from build123d import *

# Parameters (mm, degrees)
SKETCH_1_W          = 58.5
SKETCH_1_H          = 60
EXTRUDE_1_DEPTH     = 1.5
FILLET_1_R          = 2.5
CUT_EXTRUDE_1_DEPTH = 2.5


with BuildPart() as part:
    # Эскиз1 → Бобышка-Вытянуть1 (new body)
    with BuildSketch(Plane.XY):
        with Locations((29.25, 30)):
            Rectangle(SKETCH_1_W, SKETCH_1_H)
    extrude(amount=EXTRUDE_1_DEPTH)

    # Скругление1
    fillet_1_edges = [part.edges().sort_by_distance(p)[0] for p in [
        (58.5, 0, 0.75),
        (0, 0, 0.75),
    ]]
    fillet(fillet_1_edges, radius=FILLET_1_R)

    # Эскиз2 → Вырез-Вытянуть1 (cut, through all)
    with BuildSketch(Plane.XY.offset(1.5)):
        with BuildLine():
            Line((24.25, 57), (34.25, 57))
            ThreePointArc((34.25, 57), (29.25, 52), (24.25, 57))
        make_face()
    extrude(amount=-CUT_EXTRUDE_1_DEPTH, mode=Mode.SUBTRACT)


solid = part.part
Read the model definition and answer for the solid it produces. Units are mm, in the model's axes. A direction names the side the tool comes from. Coordinates: 2 decimals unless noted, no trailing zeros. Write each loop counter-clockwise with the first axis right and the second up, starting at its lowest first coordinate (ties: lowest second). Pieces come first, ordered by that corner, then holes. Notation, with made-up numbers: (-32, 87.5) -> (11, 87.5) arc R26 ccw to (11, 101.5) -> close; hole circle Ø2 at (-38.5, -25.5). An arc over 180 degrees is marked (long way). Return JSON: item names as keys, results as strings.
(1) For a pull along X with two mould halves and no side action, classify faces 3 (the flat face through (29, 57, 1)), 4 (the flat face through (58.5, 31, 1)), 5 (the flat face through (29, 60, 1)) as pulls with the +X half, pulls with the -X half, needs draft (parallel to the pull), parting line crosses it, or undercut.
Answers below:
{"face 3": "undercut", "face 4": "pulls with the +X half", "face 5": "needs draft"}
(2) Consider line 1 along Y through (x, z) = (25.5, 0.8). Determine where the line is inside the solid, lowest interval first. Write a range as from..to.
Answers below:
{"line 1": "0..53.69, 57..60"}
(3) The part is cut by section A-A on x = 29.25. Give the vertices of the cut face in (y, z), then the cut area to 3 significant figures.
Answers below:
{"outline": "(0, 0) -> (52, 0) -> (52, 1.5) -> (0, 1.5) -> close; (57, 0) -> (60, 0) -> (60, 1.5) -> (57, 1.5) -> close", "area": "82.5 mm^2"}
(4) Which of the six approach directions +Z, -Z, +X, -X, +Y, -Y give full straight-line access (tool end or side, diameter ignored) to faces 1 (the cylindrical face through (29.36, 52, 0.76)), 2 (the flat face through (29, 30, 0))?
Answers below:
{"face 1": "+Z, -Z", "face 2": "-Z, +X, -X, +Y, -Y"}
